Geometry: final body of the model. Coordinates: model frame, mm. A direction names the side the tool comes from. Coordinates: 2 decimals unless noted, no trailing zeros. Write each loop counter-clockwise with the first axis right and the second up, starting at its lowest first coordinate (ties: lowest second). Pieces come first, ordered by that corner, then holes. Notation, with made-up numbers: M 34.5,46 L 43.5,46 A16 ccw 43.5,67 Z; hole C 68,58 d10. An arc over 180 degrees is marked long. Write item = value, one per line. Start each with the question number.
Item 1: Section A-A on y = 1.25. Output: boundary loops of the cut face in (x, z).
Item 2: First-contact query: pin 1 Ø5 at (x, z) = (-9, -17) entering from +Y; pin 2 Ø5 at (x, y) = (12.5, 3) entering from -Z; pin 3 Ø4 at (x, y) = (8.5, 4.5) entering from +Z; pin 4 Ø1.8 at (x, z) = (9, 17) entering from -Y. Flat tips, straight axial feed; report the tip coordinate or a pass-through.
Item 3: Section D-D on z = 0. Output: boundary loops of the cut face in (x, y).
Item 4: Reachability of faces 1 (the cylindrical face through (-39.05, 1.97, -8.67)), 2 (the cylindrical face through (15.543, 8.93, -29.336)) from +Z, -Z, +X, -X, +Y, -Y: full face, straight path, thin tool, end or side. Return the list, or none.
Item 5: Section B-B on z = 17. Output: boundary loops of the cut face in (x, y).
Item 6: Ray query, L1, parallel to X at y = 3.25, z = 17; L2, parallel to Y at x = 34.5, z = 14; L3, parallel to Z at x = 33.5, y = 1.5. Return the intervals inside material, ascending. Write a range as [from, to].
Item 7: Section C-C on x = -32. Output: boundary loops of the cut face in (y, z), plus the area to 3 significant figures.
Item 8: Pull-direction query (X, two-part tool) for faces 3 (the cylindrical face through (-11.86, 8.93, 30.39)), 4 (the flat face through (-12, 14, 33)), 5 (the cylindrical face through (-8.93, 1.97, -18.5)); classes: +X half, -X half, draft (parallel to the pull), parting line (faces both ways), or undercut.
from build123d import *

# Parameters (mm, degrees)
SKETCH1_R           = 40
SKETCH1_R_2         = 1.5
BOSS_EXTRUDE1_DEPTH = 4
SKETCH2_R           = 2.5
BOSS_EXTRUDE2_DEPTH = 10


with BuildPart() as part:
    # Sketch1 → Boss-Extrude1 (new body)
    with BuildSketch(Plane(origin=(0, 0, 0), x_dir=(1, 0, 0), z_dir=(0, 1, 0))):
        with Locations(Location((0, 0, 0), (0, 0, 270))):
            Circle(SKETCH1_R)
        with Locations(Location((9, 17, 0), (0, 0, 270))):
            Circle(SKETCH1_R_2, mode=Mode.SUBTRACT)
        with Locations(Location((-9, 17, 0), (0, 0, 270))):
            Circle(SKETCH1_R_2, mode=Mode.SUBTRACT)
        with Locations(Location((-9, -17, 0), (0, 0, 270))):
            Circle(SKETCH1_R_2, mode=Mode.SUBTRACT)
        with Locations(Location((9, -17, 0), (0, 0, 270))):
            Circle(SKETCH1_R_2, mode=Mode.SUBTRACT)
    extrude(amount=BOSS_EXTRUDE1_DEPTH)

    # Sketch2 → Boss-Extrude2 (add)
    with BuildSketch(Plane(origin=(0, 4, 0), x_dir=(1, 0, 0), z_dir=(0, 1, 0))):
        with Locations(Location((14.791639161, 31.720772546, 0), (0, 0, 270))):
            Circle(SKETCH2_R)
        with Locations(Location((-11.970705016, -32.889241728, 0), (0, 0, 270))):
            Circle(SKETCH2_R)
    extrude(amount=BOSS_EXTRUDE2_DEPTH)


solid = part.part
Responses:
q1.outline = C 0,0 d80; hole C -9,-17 d3; hole C -9,17 d3; hole C 9,-17 d3; hole C 9,17 d3
q2.pin_1 = 4
q2.pin_2 = -38.73
q2.pin_3 = 39.46
q2.pin_4 = through
q3.outline = M -40,0 L 40,0 L 40,4 L -40,4 Z
q4.face_1 = +Y, -Y
q4.face_2 = +Y
q5.outline = M -36.21,0 L -10.5,0 L -10.5,4 L -36.21,4 Z; M -7.5,0 L 7.5,0 L 7.5,4 L -7.5,4 Z; M 10.5,0 L 36.21,0 L 36.21,4 L 10.5,4 Z
q6.L1 = [-36.21, -10.5], [-7.5, 7.5], [10.5, 36.21]
q6.L2 = [0, 4]
q6.L3 = [-21.86, 21.86]
q7.outline = M 0,-24 L 4,-24 L 4,24 L 0,24 Z
q7.area = 192 mm²
q8.face_3 = parting line
q8.face_4 = draft
q8.face_5 = undercut
